```python
from build123d import *

# Parameters (mm, degrees)
SKETCH_W        = 100
SKETCH_H        = 195
PAD_DEPTH       = 10
SKETCH001_W     = 80
SKETCH001_H     = 170
POCKET_DEPTH    = 10.001
SKETCH003_W     = 93
SKETCH003_H     = 185
POCKET001_DEPTH = 6


with BuildPart() as part:
    # Sketch → Pad (new body)
    with BuildSketch(Plane.XY):
        Rectangle(SKETCH_W, SKETCH_H)
    extrude(amount=PAD_DEPTH)

    # Sketch001 → Pocket (cut, through all)
    with BuildSketch(Plane.XY.offset(10)):
        Rectangle(SKETCH001_W, SKETCH001_H)
    extrude(amount=-POCKET_DEPTH, mode=Mode.SUBTRACT)

    # Sketch003 → Pocket001 (cut)
    with BuildSketch(Plane.XY.offset(10)):
        with Locations((0, -0.235933)):
            Rectangle(SKETCH003_W, SKETCH003_H)
    extrude(amount=-POCKET001_DEPTH, mode=Mode.SUBTRACT)


solid = part.part
```
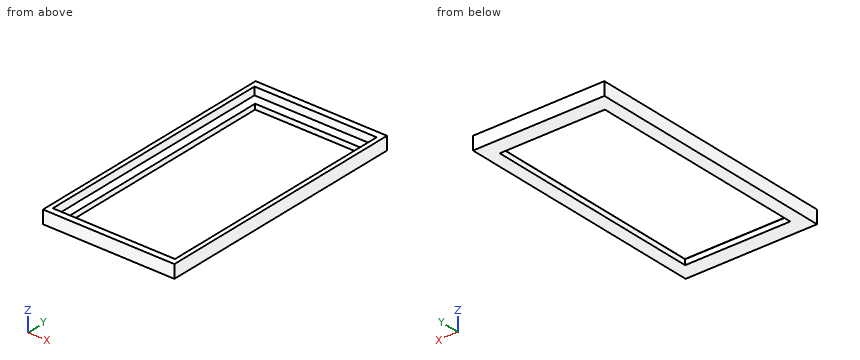
Verification items for the finished model (mm, model axes). Give positions to 0.01 mm unless a question says otherwise; leave off trailing zeros. Order: outer loops, then holes, each group sorted by start corner. A loop starts at its lowest first (then second) coordinate and runs counter-clockwise, first axis right, second up. Notation, with made-up numbers: (87, 19) -> (100, 19) arc R19 cw to (100, 44) -> close; hole circle Ø1 at (-14.75, -13). An arc over 180 degrees is marked (long way). Use a Markdown table: item, result.
1) Depth check by flat-ended pin: pin 1 Ø12 at (x, y) = (-31, 14.5) entering from -Z. Enter the tip coordinate at first touch or a pass-through.
Results:
| item | result |
|---|---|
| pin 1 | through |
2) Material ranges on probe 1 along X at (y, z) = (10.5, 7.25); probe 2 along Y at (x, z) = (-1.5, 2); probe 3 along Y at (x, z) = (-3.5, 9), recorded low to high.
Results:
| item | result |
|---|---|
| probe 1 | -50 to -46.5, 46.5 to 50 |
| probe 2 | -97.5 to -85, 85 to 97.5 |
| probe 3 | -97.5 to -92.74, 92.26 to 97.5 |
3) Section check B-B, the plane x = -11.5. Record the boundary of the cut face in (y, z).
Results:
| item | result |
|---|---|
| outline | (-97.5, 0) -> (-85, 0) -> (-85, 4) -> (-92.74, 4) -> (-92.74, 10) -> (-97.5, 10) -> close; (85, 0) -> (97.5, 0) -> (97.5, 10) -> (92.26, 10) -> (92.26, 4) -> (85, 4) -> close |
4) Section check C-C, the plane z = 1.75. Record the boundary of the cut face in (x, y), then the cut area to 3 significant figures.
Results:
| item | result |
|---|---|
| outline | (-50, -97.5) -> (50, -97.5) -> (50, 97.5) -> (-50, 97.5) -> close; hole (-40, -85) -> (40, -85) -> (40, 85) -> (-40, 85) -> close |
| area | 5,900 mm² |
5) Section check A-A, the plane y = 4.5. Record the boundary of the cut face in (x, z), then the cut area to 3 significant figures.
Results:
| item | result |
|---|---|
| outline | (-50, 0) -> (-40, 0) -> (-40, 4) -> (-46.5, 4) -> (-46.5, 10) -> (-50, 10) -> close; (40, 0) -> (50, 0) -> (50, 10) -> (46.5, 10) -> (46.5, 4) -> (40, 4) -> close |
| area | 122 mm² |
